from build123d import *

# Parameters (mm, degrees)
TUBE_R          = 15
TUBE_R_2        = 1.2
TUBE_DEPTH      = 25
CHAMFER_SIZE    = 6
CHAMFER001_SIZE = 8
FILLET_R        = 40


with BuildPart() as part:
    # Tube → Tube (new body)
    with BuildSketch(Plane.XY):
        Circle(TUBE_R)
        Circle(TUBE_R_2, mode=Mode.SUBTRACT)
    extrude(amount=TUBE_DEPTH)

    # Chamfer
    chamfer_edges = [part.edges().sort_by_distance(p)[0] for p in [
        (-15, 0, 25),
    ]]
    chamfer(chamfer_edges, length=CHAMFER_SIZE)

    # Chamfer001
    chamfer001_edges = [part.edges().sort_by_distance(p)[0] for p in [
        (-15, 0, 19),
    ]]
    chamfer(chamfer001_edges, length=CHAMFER001_SIZE)

    # Fillet
    fillet_edges = [part.edges().sort_by_distance(p)[0] for p in [
        (-14.999996, 0, 11),
    ]]
    fillet(fillet_edges, radius=FILLET_R)


with BuildPart() as part_1:
    # Fillet placement: moved
    add(part.part.moved(Location((0, 0, 60))))


solid = part_1.part
CAD build for the part. Positions are in the model's coordinates, mm. Round coordinates to 2 decimals unless told otherwise and drop trailing zeros.
(1) Two-plate mould, pull along Y, no slides. Class faces 1 (the cylindrical face through (-14.985, 0.66, 61.501)), 2 (the flat face through (3, 0, 60)), 3 (the cylindrical face through (0.65, 1.01, 72.32)): +Y half, -Y half, draft (parallel to the pull), parting line (faces both ways), or undercut.
(2) Drop flat-ended pins along their axis: pin 1 (10 mm diameter, centred on x = 9.5, y = -8, fed in from +Z); pin 2 (8 mm diameter, centred on y = -9, z = 62.5, fed in from -X); pin 3 (5 mm diameter, centred on y = -9.5, z = 78, fed in from +X); pin 4 (5 mm diameter, centred on x = -6, z = 69, fed in from +Y). Give the stop position or say it passes through.
(3) Wall check: line 1 along Y through (x, z) = (0, 73.75); line 2 along Y through (x, z) = (0, 78.5); line 3 along X through (y, z) = (1, 72.25). Give the ranges that are in metal, low to high.
Findings below:
1. face 1: parting line
1. face 2: draft
1. face 3: undercut
2. pin 1: stops at z = 85
2. pin 2: stops at x = -14.14
2. pin 3: stops at x = 10.22
2. pin 4: stops at y = 14.22
3. line 1: y = -13.54 to -1.2, 1.2 to 13.54
3. line 2: y = -11.89 to -1.2, 1.2 to 11.89
3. line 3: x = -13.89 to -0.66, 0.66 to 13.89
